```python
from build123d import *

# Parameters (mm, degrees)
SALIENTE_EXTRUIR1_DEPTH = 2
CROQUIS4_W              = 53.035898385
CROQUIS4_H              = 5
SALIENTE_EXTRUIR2_DEPTH = 2
CROQUIS5_W              = 53.035898385
CROQUIS5_H              = 5
SALIENTE_EXTRUIR3_DEPTH = 2
CROQUIS6_W              = 11.5
CROQUIS6_H              = 10.828307393
CROQUIS6_W_2            = 27
CROQUIS6_H_2            = 3
CORTAR_EXTRUIR1_DEPTH   = 10


with BuildPart() as part:
    # Croquis3 → Saliente-Extruir1 (new body)
    with BuildSketch(Plane(origin=(0, 0, 0), x_dir=(1, 0, 0), z_dir=(0, 1, 0))):
        Polygon((10.064101615, 59.412461498), (60.135898385, 59.412461498), (63.1, 59.412461498), (63.1, 56.448359883), (63.1, 48.584154105), (59.1, 48.584154105), (59.1, 23.412461498), (49.6, 23.412461498), (49.6, 3.412461498), (20.6, 3.412461498), (20.6, 23.412461498), (7.1, 23.412461498), (7.1, 56.448359883), (7.1, 59.412461498), align=None)
    extrude(amount=SALIENTE_EXTRUIR1_DEPTH)

    # Croquis4 → Saliente-Extruir2 (add)
    with BuildSketch(Plane.ZY.offset(-20.6)):
        with Locations((-29.930410691, -0.5)):
            Rectangle(CROQUIS4_W, CROQUIS4_H)
    extrude(amount=SALIENTE_EXTRUIR2_DEPTH)

    # Croquis5 → Saliente-Extruir3 (add)
    with BuildSketch(Plane(origin=(49.6, 0, 0), x_dir=(0, 0, -1), z_dir=(1, 0, 0))):
        with Locations((29.930410691, -0.5)):
            Rectangle(CROQUIS5_W, CROQUIS5_H)
    extrude(amount=SALIENTE_EXTRUIR3_DEPTH)

    # Croquis6 → Cortar-Extruir1 (cut)
    with BuildSketch(Plane(origin=(0, 2, 0), x_dir=(1, 0, 0), z_dir=(0, 1, 0))):
        with Locations((12.85, 53.998307802)):
            Rectangle(CROQUIS6_W, CROQUIS6_H)
        with Locations((35.1, 4.912461498)):
            Rectangle(CROQUIS6_W_2, CROQUIS6_H_2)
    extrude(amount=-CORTAR_EXTRUIR1_DEPTH, mode=Mode.SUBTRACT)


solid = part.part
```
Could you check a few things on this model? Use its own coordinates, in mm. A direction names the side the tool comes from. Round coordinates to 2 decimals unless told otherwise and drop trailing zeros. Loops run counter-clockwise (first coordinate to the right, second up) from the corner with the lowest first, then second, coordinate; pieces in that order, holes last. Notation, with made-up numbers: (39.5, -11.5) - (98.5, -11.5) arc R11 ccw to (98.5, -2.5) - close; hole circle Ø3 at (-6.75, -13). An arc over 180 degrees is marked (long way). Answer as CSV lines item,"result".
1. We'd pull the mould along X, two halves only. Please class faces 5 (the face through (13, 1, -23.412)), 6 (the face through (21.6, 1, -5)), 7 (the face through (63.1, 1, -54)): +X half, -X half, draft (parallel to the pull), parting line (faces both ways), or undercut.
Filled in:
face 5,"draft"
face 6,"undercut"
face 7,"+X half"
2. I want a section at C-C on x = 13.5. List the corners of the cut face in (y, z) for me.
Filled in:
outline,"(0, -48.58) - (2, -48.58) - (2, -23.41) - (0, -23.41) - close"
3. On a 3-axis mill with a long thin cutter (end or side, diameter ignored), from which of +Z, -Z, +X, -X, +Y, -Y can I reach the whole of each face in a straight line? I mean faces 1 (the face through (13, 1, -48.584)), 2 (the face through (48.6, 1, -5)), 3 (the face through (20.6, -1, -30)), 4 (the face through (13, 0, -36)). Say none if no direction works.
Filled in:
face 1,"-Z, -X, +Y, -Y"
face 2,"+Z, +Y, -Y"
face 3,"+Z, -Z, -Y"
face 4,"+Z, -Z, -X, -Y"
4. I want a section at B-B on z = -16. List the corners of the cut face in (x, y) for me, then the cut area to 3 significant figures.
Filled in:
outline,"(18.6, -3) - (20.6, -3) - (20.6, 0) - (49.6, 0) - (49.6, -3) - (51.6, -3) - (51.6, 2) - (18.6, 2) - close"
area,"78.0 mm^2"
5. I want a section at A-A on y = -1.65. List the corners of the cut face in (x, z) for me, then the cut area to 3 significant figures.
Filled in:
outline,"(18.6, -56.45) - (20.6, -56.45) - (20.6, -3.41) - (18.6, -3.41) - close; (49.6, -56.45) - (51.6, -56.45) - (51.6, -3.41) - (49.6, -3.41) - close"
area,"212 mm^2"
6. Please list where these lines run through material, in increasing order: line 1 along X through (y, z) = (-0.55, -27); line 2 along X through (y, z) = (1.2, -5.5); line 3 along Z through (x, y) = (45, 1.3). Write a range as [from, to].
Filled in:
line 1,"x = [18.6, 20.6], [49.6, 51.6]"
line 2,"x = [18.6, 21.6], [48.6, 51.6]"
line 3,"z = [-59.41, -6.41]"
7. I want a section at D-D on z = -52.5. List the corners of the cut face in (x, y) for me, then the cut area to 3 significant figures.
Filled in:
outline,"(18.6, -3) - (20.6, -3) - (20.6, 0) - (49.6, 0) - (49.6, -3) - (51.6, -3) - (51.6, 0) - (63.1, 0) - (63.1, 2) - (18.6, 2) - close"
area,"101 mm^2"
8. For pin 1 Ø3 at (y, z) = (0.5, -29.5) entering from +X; pin 2 Ø13.5 at (x, z) = (31.5, -22) entering from -Y; pin 3 Ø1 at (y, z) = (0.5, -5.5) entering from +X, each with a flat end and sliding along its axis, tell me the tip position at first contact or that it passes through.
Filled in:
pin 1,"stops at x = 59.1"
pin 2,"stops at y = 0"
pin 3,"stops at x = 51.6"
